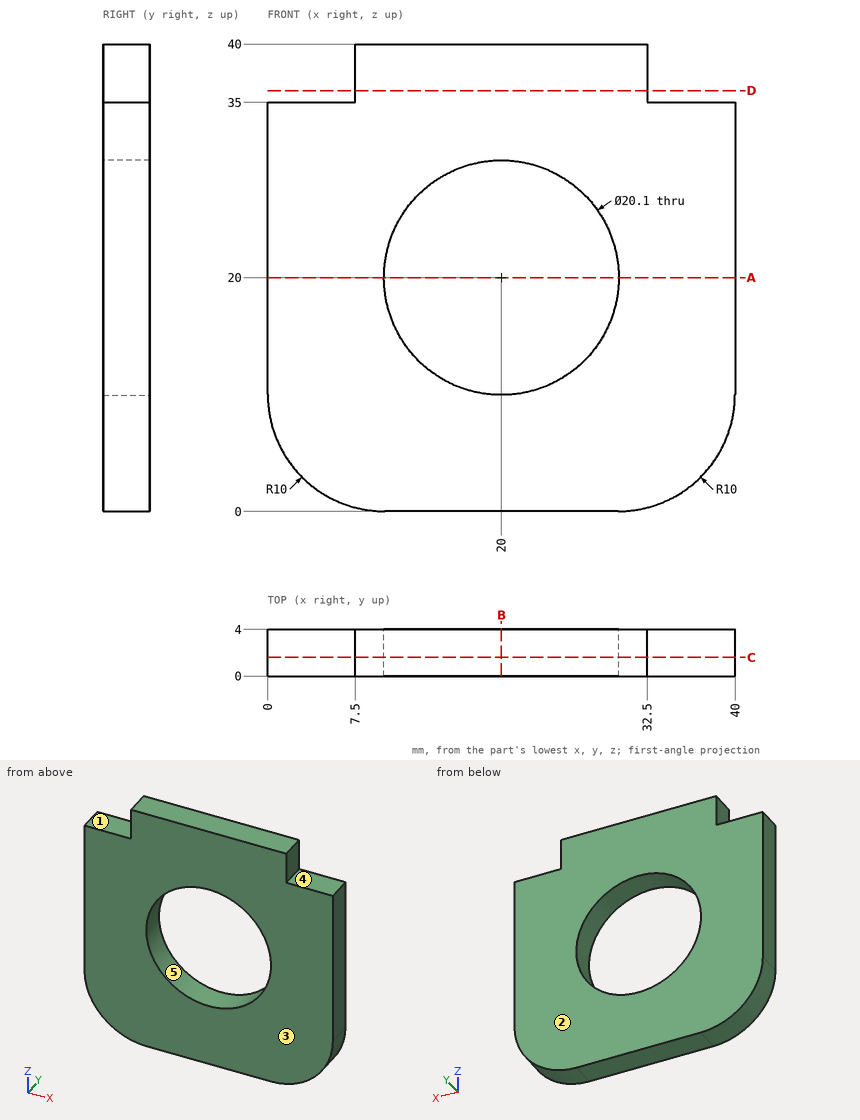
Answer from the drawing. Dimensions are ordinates in mm from the lowest x, y and z of the part. A direction names the side the tool comes from. Give positions to 0.01 mm unless a question says otherwise; leave off trailing zeros. Loops run counter-clockwise (first coordinate to the right, second up) from the corner with the lowest first, then second, coordinate; pieces in that order, holes last. Notation, with made-up numbers: (-6, -23.5) - (29, -23.5) arc R11 cw to (29, -9.5) - close; hole circle Ø7 at (27.5, 82.25). An arc over 180 degrees is marked (long way). Answer as a JSON object with one key per item and string values.
1. Flat-ended cylindrical pins translate along their axes: pin 1 Ø2 at (y, z) = (2.5, 37) entering from +X; pin 2 Ø2 at (x, y) = (4.5, 3) entering from +Z. Find the tip coordinate at first contact, or state that the pin passes through.
Determined:
{"pin 1": "x = 32.5", "pin 2": "z = 35"}
2. For the marked faces 1 and 2, determine the directions among +Z, -Z, +X, -X, +Y, -Y from which every point of the face is accessible in a straight line to the end or side of a thin tool.
Determined:
{"face 1": "+Z, -X, +Y, -Y", "face 2": "+Z, -Z, +X, -X, +Y"}
3. A cutting plane is placed at C-C (y = 1.6). Write down the section's boundary in (x, z).
Determined:
{"outline": "(0, 10) arc R10 ccw to (10, 0) - (30, 0) arc R10 ccw to (40, 10) - (40, 35) - (32.5, 35) - (32.5, 40) - (7.5, 40) - (7.5, 35) - (0, 35) - close; hole circle Ø20.1 at (20, 20)"}
4. A cutting plane is placed at D-D (z = 36). Write down the section's boundary in (x, y).
Determined:
{"outline": "(7.5, 0) - (32.5, 0) - (32.5, 4) - (7.5, 4) - close"}
5. For a pull along Z with two mould halves and no side action, classify the marked faces 3, 4 and 5 as pulls with the +Z half, pulls with the -Z half, needs draft (parallel to the pull), parting line crosses it, or undercut.
Determined:
{"face 3": "needs draft", "face 4": "pulls with the +Z half", "face 5": "undercut"}
6. A cutting plane is placed at A-A (z = 20). Write down the section's boundary in (x, y).
Determined:
{"outline": "(0, 0) - (9.95, 0) - (9.95, 4) - (0, 4) - close; (30.05, 0) - (40, 0) - (40, 4) - (30.05, 4) - close"}
7. A cutting plane is placed at B-B (x = 20). Write down the section's boundary in (y, z).
Determined:
{"outline": "(0, 0) - (4, 0) - (4, 9.95) - (0, 9.95) - close; (0, 30.05) - (4, 30.05) - (4, 40) - (0, 40) - close"}
8. Find the intervals of material crossed by L1, parallel to Z at x = 19, y = 0.8; L2, parallel to X at y = 2.55, z = 20; L3, parallel to X at y = 2.35, z = 14, in increasing order. Write a range as [from, to].
Determined:
{"L1": "[0, 10], [30, 40]", "L2": "[0, 9.95], [30.05, 40]", "L3": "[0, 11.94], [28.06, 40]"}
